Here's how the part is built. I have some questions about the finished solid (model axes, mm). Round coordinates to 2 decimals unless told otherwise and drop trailing zeros. Order: outer loops, then holes, each group sorted by start corner. A loop starts at its lowest first (then second) coordinate and runs counter-clockwise, first axis right, second up. Notation, with made-up numbers: (6, -31) -> (59, -31) arc R8 ccw to (59, -23) -> close; hole circle Ø5 at (-7, 86). An arc over 180 degrees is marked (long way). One line per item, written item: value.
Autodesk Inventor part; units mm, degrees
ref_plane "YZ Plane" through (0, 0, 0) normal (1, 0, 0) x (0, 1, 0)
ref_plane "XZ Plane" through (0, 0, 0) normal (0, 1, 0) x (-1, 0, 0)
ref_plane "XY Plane" through (0, 0, 0) normal (0, 0, 1) x (1, 0, 0)
sketch "Sketch7" plane through (0, 0, 0) normal (0, 0, 1) x (1, 0, 0)
  circle A0 centre (-231.5775, 231.5775) radius 3.4
  line L0 (-231.5775, 203.2932) -> (-203.2932, 231.5775)
  line L1 (-203.2932, 231.5775) -> (-231.5775, 259.8617)
  line L2 (-231.5775, 259.8617) -> (-259.8617, 231.5775)
  line L3 (-259.8617, 231.5775) -> (-231.5775, 203.2932)
  line L4 (-231.5775, 203.2932) -> (-231.5775, 259.8617) construction
  line L5 (-203.2932, 231.5775) -> (-259.8617, 231.5775) construction
  line L6 (-231.5775, 203.2932) -> (-191.5775, 203.2932) construction
  arc A1 (289.9795, 47.2262) -> (285.9788, 67.3391) centre (0, 0) ccw construction
  arc A2 (295.9015, 48.1906) -> (291.8191, 68.7143) centre (0, 0) ccw
  arc A3 (284.0576, 46.2617) -> (280.1386, 65.9639) centre (0, 0) ccw
  arc A4 (284.0576, 46.2617) -> (295.9015, 48.1906) centre (289.9795, 47.2262) ccw
  arc A5 (291.8191, 68.7143) -> (280.1386, 65.9639) centre (285.9788, 67.3391) ccw
  line L7 (0, 0) -> (289.9795, 47.2262) construction
  line L8 (0, 0) -> (293.8, 0) construction
  line L9 (0, 0) -> (285.9788, 67.3391) construction
  circle A6 centre (0, 0) radius 307.5
  circle A7 centre (0, 0) radius 282.5
  line L10 (-203.2932, 231.5775) -> (-185.1143, 213.3986)
  line L11 (-231.5775, 203.2932) -> (-213.3986, 185.1143)
  line L12 (-307.5, 0) -> (0, 0)
  line L13 (0, 0) -> (307.5, 0)
  line L14 (-231.5775, -203.2932) -> (-259.8617, -231.5775)
  line L15 (-259.8617, -231.5775) -> (-231.5775, -259.8617)
  circle A8 centre (-231.5775, -231.5775) radius 3.4
  line L16 (-231.5775, -259.8617) -> (-203.2932, -231.5775)
  line L17 (-203.2932, -231.5775) -> (-231.5775, -203.2932)
  line L18 (-203.2932, -231.5775) -> (-185.1143, -213.3986)
  line L19 (-231.5775, -203.2932) -> (-213.3986, -185.1143)
  line L20 (203.2932, -231.5775) -> (231.5775, -259.8617)
  line L21 (231.5775, -259.8617) -> (259.8617, -231.5775)
  circle A9 centre (231.5775, -231.5775) radius 3.4
  line L22 (259.8617, -231.5775) -> (231.5775, -203.2932)
  line L23 (231.5775, -203.2932) -> (203.2932, -231.5775)
  line L24 (231.5775, -203.2932) -> (213.3986, -185.1143)
  line L25 (203.2932, -231.5775) -> (185.1143, -213.3986)
  line L26 (231.5775, 203.2932) -> (259.8617, 231.5775)
  line L27 (259.8617, 231.5775) -> (231.5775, 259.8617)
  circle A10 centre (231.5775, 231.5775) radius 3.4
  line L28 (231.5775, 259.8617) -> (203.2932, 231.5775)
  line L29 (203.2932, 231.5775) -> (231.5775, 203.2932)
  line L30 (203.2932, 231.5775) -> (185.1143, 213.3986)
  line L31 (231.5775, 203.2932) -> (213.3986, 185.1143)
  arc A11 (254.9356, 157.7589) -> (243.3099, 175.158) centre (0, 0) ccw
  arc A12 (243.3099, 175.158) -> (233.571, 168.1471) centre (238.4404, 171.6526) ccw
  arc A13 (244.7314, 151.4444) -> (233.571, 168.1471) centre (0, 0) ccw
  arc A14 (244.7314, 151.4444) -> (254.9356, 157.7589) centre (249.8335, 154.6017) ccw
  arc A15 (175.158, 243.3099) -> (157.7589, 254.9356) centre (0, 0) ccw
  arc A16 (157.7589, 254.9356) -> (151.4444, 244.7314) centre (154.6017, 249.8335) ccw
  arc A17 (168.1471, 233.571) -> (151.4444, 244.7314) centre (0, 0) ccw
  arc A18 (168.1471, 233.571) -> (175.158, 243.3099) centre (171.6526, 238.4404) ccw
  arc A19 (68.7143, 291.8191) -> (48.1906, 295.9015) centre (0, 0) ccw
  arc A20 (48.1906, 295.9015) -> (46.2617, 284.0576) centre (47.2262, 289.9795) ccw
  arc A21 (65.9639, 280.1386) -> (46.2617, 284.0576) centre (0, 0) ccw
  arc A22 (65.9639, 280.1386) -> (68.7143, 291.8191) centre (67.3391, 285.9788) ccw
  arc A23 (-48.1906, 295.9015) -> (-68.7143, 291.8191) centre (0, 0) ccw
  arc A24 (-68.7143, 291.8191) -> (-65.9639, 280.1386) centre (-67.3391, 285.9788) ccw
  arc A25 (-46.2617, 284.0576) -> (-65.9639, 280.1386) centre (0, 0) ccw
  arc A26 (-46.2617, 284.0576) -> (-48.1906, 295.9015) centre (-47.2262, 289.9795) ccw
  arc A27 (-157.7589, 254.9356) -> (-175.158, 243.3099) centre (0, 0) ccw
  arc A28 (-175.158, 243.3099) -> (-168.1471, 233.571) centre (-171.6526, 238.4404) ccw
  arc A29 (-151.4444, 244.7314) -> (-168.1471, 233.571) centre (0, 0) ccw
  arc A30 (-151.4444, 244.7314) -> (-157.7589, 254.9356) centre (-154.6017, 249.8335) ccw
  arc A31 (-243.3099, 175.158) -> (-254.9356, 157.7589) centre (0, 0) ccw
  arc A32 (-254.9356, 157.7589) -> (-244.7314, 151.4444) centre (-249.8335, 154.6017) ccw
  arc A33 (-233.571, 168.1471) -> (-244.7314, 151.4444) centre (0, 0) ccw
  arc A34 (-233.571, 168.1471) -> (-243.3099, 175.158) centre (-238.4404, 171.6526) ccw
  arc A35 (-291.8191, 68.7143) -> (-295.9015, 48.1906) centre (0, 0) ccw
  arc A36 (-295.9015, 48.1906) -> (-284.0576, 46.2617) centre (-289.9795, 47.2262) ccw
  arc A37 (-280.1386, 65.9639) -> (-284.0576, 46.2617) centre (0, 0) ccw
  arc A38 (-280.1386, 65.9639) -> (-291.8191, 68.7143) centre (-285.9788, 67.3391) ccw
  arc A39 (-295.9015, -48.1906) -> (-291.8191, -68.7143) centre (0, 0) ccw
  arc A40 (-291.8191, -68.7143) -> (-280.1386, -65.9639) centre (-285.9788, -67.3391) ccw
  arc A41 (-284.0576, -46.2617) -> (-280.1386, -65.9639) centre (0, 0) ccw
  arc A42 (-284.0576, -46.2617) -> (-295.9015, -48.1906) centre (-289.9795, -47.2262) ccw
  arc A43 (-254.9356, -157.7589) -> (-243.3099, -175.158) centre (0, 0) ccw
  arc A44 (-243.3099, -175.158) -> (-233.571, -168.1471) centre (-238.4404, -171.6526) ccw
  arc A45 (-244.7314, -151.4444) -> (-233.571, -168.1471) centre (0, 0) ccw
  arc A46 (-244.7314, -151.4444) -> (-254.9356, -157.7589) centre (-249.8335, -154.6017) ccw
  arc A47 (-175.158, -243.3099) -> (-157.7589, -254.9356) centre (0, 0) ccw
  arc A48 (-157.7589, -254.9356) -> (-151.4444, -244.7314) centre (-154.6017, -249.8335) ccw
  arc A49 (-168.1471, -233.571) -> (-151.4444, -244.7314) centre (0, 0) ccw
  arc A50 (-168.1471, -233.571) -> (-175.158, -243.3099) centre (-171.6526, -238.4404) ccw
  arc A51 (-68.7143, -291.8191) -> (-48.1906, -295.9015) centre (0, 0) ccw
  arc A52 (-48.1906, -295.9015) -> (-46.2617, -284.0576) centre (-47.2262, -289.9795) ccw
  arc A53 (-65.9639, -280.1386) -> (-46.2617, -284.0576) centre (0, 0) ccw
  arc A54 (-65.9639, -280.1386) -> (-68.7143, -291.8191) centre (-67.3391, -285.9788) ccw
  arc A55 (48.1906, -295.9015) -> (68.7143, -291.8191) centre (0, 0) ccw
  arc A56 (68.7143, -291.8191) -> (65.9639, -280.1386) centre (67.3391, -285.9788) ccw
  arc A57 (46.2617, -284.0576) -> (65.9639, -280.1386) centre (0, 0) ccw
  arc A58 (46.2617, -284.0576) -> (48.1906, -295.9015) centre (47.2262, -289.9795) ccw
  arc A59 (157.7589, -254.9356) -> (175.158, -243.3099) centre (0, 0) ccw
  arc A60 (175.158, -243.3099) -> (168.1471, -233.571) centre (171.6526, -238.4404) ccw
  arc A61 (151.4444, -244.7314) -> (168.1471, -233.571) centre (0, 0) ccw
  arc A62 (151.4444, -244.7314) -> (157.7589, -254.9356) centre (154.6017, -249.8335) ccw
  arc A63 (243.3099, -175.158) -> (254.9356, -157.7589) centre (0, 0) ccw
  arc A64 (254.9356, -157.7589) -> (244.7314, -151.4444) centre (249.8335, -154.6017) ccw
  arc A65 (233.571, -168.1471) -> (244.7314, -151.4444) centre (0, 0) ccw
  arc A66 (233.571, -168.1471) -> (243.3099, -175.158) centre (238.4404, -171.6526) ccw
  arc A67 (291.8191, -68.7143) -> (295.9015, -48.1906) centre (0, 0) ccw
  arc A68 (295.9015, -48.1906) -> (284.0576, -46.2617) centre (289.9795, -47.2262) ccw
  arc A69 (280.1386, -65.9639) -> (284.0576, -46.2617) centre (0, 0) ccw
  arc A70 (280.1386, -65.9639) -> (291.8191, -68.7143) centre (285.9788, -67.3391) ccw
  circle A71 centre (327.5, 0) radius 20
  line L32 (345.0573, 9.5783) -> (269.9427, 147.2656)
  point P0 (-202.8328, 231.1171)
  point P1 (-231.1171, 202.8328)
  point P2 (-282.5, 0)
  point P3 (282.5, 0)
  point P4 (231.1171, 202.8328)
  point P5 (202.8328, 231.1171)
  point P6 (307.5, 0)
  dimension "d173" = 40
  dimension "d131" = 6.8
  dimension "d132" = 231.5775
  dimension "d133" = 231.5775
  dimension "d135" = 45
  dimension "d137" = 40
  dimension "d138" = 40
  dimension "d144" = 293.8
  dimension "d145" = 9.25
  dimension "d146" = 4
  dimension "d147" = 12
  dimension "d148" = 615
  dimension "d149" = 565
  dimension "d152" = 360
  dimension "d156" = 360
  dimension "d174" = 0
  dimension "d175" = 327.5
extrude "Extrusion11" add sketch "Sketch7" against normal blind 10 contours L3 L2 L1 L0 | L0 A6 L11 | L0 L10 A6 | A6 L10 A7 L11 | L11 A7 L12 A6 | A6 L30 A7 L10 | L30 L29 A6 | A6 L31 A7 L30 | L29 L31 A6 | L29 L28 L27 L26 | A6 L13 A7 L31
fillet "Fillet4" radius 4 8 edges at (-231.1171, 202.8328, -5) (-259.8617, 231.5775, -5) (-202.8328, 231.1171, -5) (-231.5775, 259.8617, -5) (231.5775, 259.8617, -5) (259.8617, 231.5775, -5) (202.8328, 231.1171, -5) (231.1171, 202.8328, -5)
extrude "Extrusion13" add sketch "Sketch7" against normal blind 5 contours L32 A71 A6 | A71
hole "Hole5" at (0, 0, 0) at (327.5, 0, 0) direction (0, 0, -1) diameter 6 end through all
equation "\"bar_screw_hole_diam\" = 6.8"
equation "\"foot_length\" = 14"
equation "\"rim_diam\" = 605"
equation "\"tube_inner_diam\" = 541"
equation "\"tube_outer_diam\" = 561"
equation "\"ring_delta\" = 2"
equation "\"bar_delta\" = 5"
equation "\"bar_circle_diam\" = 655"
equation "\"ring_inner_diam\" = 565"
equation "\"ring_outer_diam\" = 615"
equation "\"slot_angle\" = 9.25deg"
equation "\"slot_diam\" = 12"
equation "\"slots_circle_diam\" = 587.6"
equation "\"foot_screw_diam\" = 6"
equation "\"bar_fillet\" = 4"
properties part number "half_ring_1" material "Aluminum 6061"
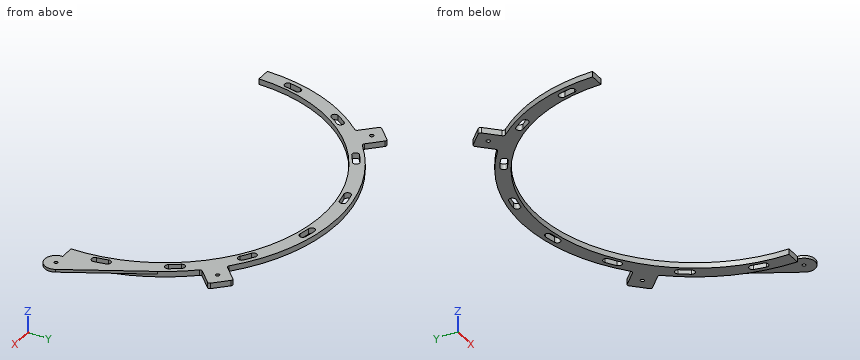
Q1. I want a section at A-A on x = 0. Write out the boundary of the cut face in (y, z), then the cut area to 3 significant figures.
Answers:
outline: (282.5, -10) -> (307.5, -10) -> (307.5, 0) -> (282.5, 0) -> close
area: 250 mm2
Q2. I want a section at C-C on x = 98. Write out the boundary of the cut face in (y, z).
Answers:
outline: (264.96, -10) -> (291.47, -10) -> (291.47, 0) -> (264.96, 0) -> close
Q3. I want a section at B-B on z = -7.5. Give the number of separate pieces and of enclosed holes in the cut face, then the cut area to 3 significant figures.
Answers:
separate pieces: 1
enclosed holes: 10
area: 23,400 mm2
Q4. For P1, Ø6, axis at y = 60, z = -7, coming from the -X side; P2, Ø1, axis at y = 178.5, z = -4.5, coming from the +X side; P3, Ø6, axis at x = -123.5, z = -5, coming from the +Y side, each with a flat end and sliding along its axis, tell me the tip position at first contact or that it passes through.
Answers:
P1: x = -302.17
P2: x = 250.74
P3: y = 282.91
Q5. I need wall thicknesses on line 1 along X through (y, z) = (2, -1); line 2 along X through (y, z) = (174.5, -2); line 3 along X through (y, z) = (71.5, -4). Which ranges of each line are inside material? Lowest first, please.
Answers:
line 1: -307.49 to -282.49, 282.49 to 325.26, 329.74 to 347.4
line 2: -253.19 to -243.78, -233.16 to -222.16, 222.16 to 233.16, 243.78 to 253.19
line 3: -299.07 to -290.3, -281.66 to -273.3, 273.3 to 281.66, 290.3 to 311.28
